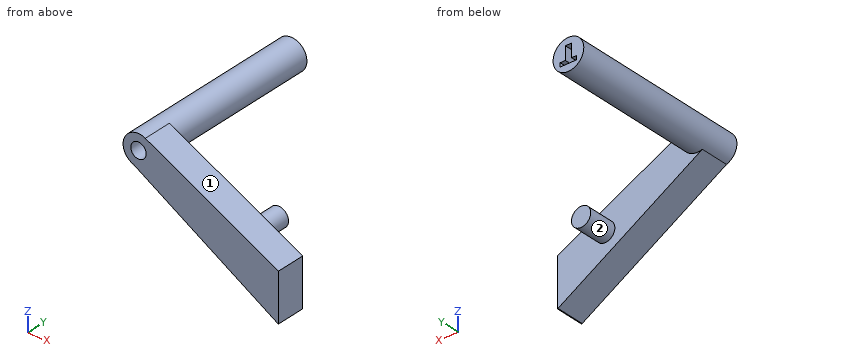
```python
from build123d import *

# Parameters (mm, degrees)
SKETCH1_R           = 8
BOSS_EXTRUDE1_DEPTH = 95
SKETCH2_R           = 4
CUT_EXTRUDE1_DEPTH  = 45
SKETCH3_W           = 8.60885167
SKETCH3_H           = 2.035138461
SKETCH3_W_2         = 3.196177608
SKETCH3_H_2         = 6.875388446
CUT_EXTRUDE2_DEPTH  = 40
BOSS_EXTRUDE2_DEPTH = 15
SKETCH5_R           = 5
BOSS_EXTRUDE3_DEPTH = 15


with BuildPart() as part:
    # Sketch1 → Boss-Extrude1 (new body)
    with BuildSketch(Plane(origin=(0, 0, 0), x_dir=(1, 0, 0), z_dir=(0, 1, 0))):
        with Locations(Location((0, 0, 0), (0, 0, 270))):
            Circle(SKETCH1_R)
    extrude(amount=BOSS_EXTRUDE1_DEPTH)

    # Sketch2 → Cut-Extrude1 (cut)
    with BuildSketch(Plane.XZ):
        with Locations(Location((0, 0, 0), (0, 0, 270))):
            Circle(SKETCH2_R)
    extrude(amount=-CUT_EXTRUDE1_DEPTH, mode=Mode.SUBTRACT)

    # Sketch3 → Cut-Extrude2 (cut)
    with BuildSketch(Plane(origin=(0, 95, 0), x_dir=(1, 0, 0), z_dir=(0, 1, 0))):
        with Locations((0, 3.24887213)):
            Rectangle(SKETCH3_W, SKETCH3_H)
        with Locations((0, -1.206391324)):
            Rectangle(SKETCH3_W_2, SKETCH3_H_2)
    extrude(amount=-CUT_EXTRUDE2_DEPTH, mode=Mode.SUBTRACT)

    # Sketch4 → Boss-Extrude2 (add)
    with BuildSketch(Plane.XZ):
        with BuildLine():
            ThreePointArc((72.61474538, -52.266719107), (72.807969556, -52.302734502), (73.001736138, -52.33570725))
            Line((73.001736138, -52.33570725), (73.001736138, -27.496744571))
            Line((73.001736138, -27.496744571), (3.57279106, 7.157874268))
            ThreePointArc((3.57279106, 7.157874268), (7.382913261, -3.081004996), (-2.575137965, -7.574210484))
            Line((-2.575137965, -7.574210484), (72.61474538, -52.266719107))
        make_face()
    extrude(amount=-BOSS_EXTRUDE2_DEPTH)

    # Sketch5 → Boss-Extrude3 (add)
    with BuildSketch(Plane(origin=(0, 15, 0), x_dir=(1, 0, 0), z_dir=(0, 1, 0))):
        with Locations(Location((48.001736138, 26.246610631, 0), (0, 0, 90))):
            Circle(SKETCH5_R)
    extrude(amount=BOSS_EXTRUDE3_DEPTH)

    # Sketch9 → Cut-Revolve2 (revolve, cut)
    with BuildSketch(Plane(origin=(0, 0, 0), x_dir=(0.6901743919423456, 0, -0.7236430810192366), z_dir=(-0.7236430810192366, 0, -0.6901743919423456)), mode=Mode.PRIVATE) as cut_revolve2_sk:
        Polygon((-4, -45), (0, -45), (0, -51.92820323), align=None)
    revolve(cut_revolve2_sk.sketch.rotate(Axis((0, 45, 0), (0, 1, 0)), 242.42131363), axis=Axis((0, 45, 0), (0, 1, 0)), mode=Mode.SUBTRACT)


solid = part.part
```
Geometry check sheet. Reference: the model listing, model coordinates, mm. Face numbers are marked on the shaded views. A direction names the side the tool comes from. Give positions to 0.01 mm unless a question says otherwise; leave off trailing zeros. Write each loop counter-clockwise with the first axis right and the second up, starting at its lowest first coordinate (ties: lowest second). Pieces come first, ordered by that corner, then holes. Notation, with made-up numbers: (38.25, -19.75) - (80.25, -19.75) arc R13 cw to (80.25, -1.75) - close; hole circle Ø9 at (85.5, 71.25). An arc over 180 degrees is marked (long way). Use a Markdown table: item, result.
Q1. Section check C-C, the plane x = 28.5. Enter the section's corners in (y, z), then the cut area to 3 significant figures.
Computed:
| item | result |
|---|---|
| outline | (0, -26.05) - (15, -26.05) - (15, -5.28) - (0, -5.28) - close |
| area | 311 mm² |
Q2. Go/stop test with flat-tipped pins: P1, Ø2, axis at x = 38.5, z = -11.5, coming from the +Y side; P2, Ø11, axis at x = 46, z = -27, coming from the +Y side; P3, Ø1.6, axis at y = 71, z = -3, coming from the -X side. Record where each tip stops, or that it passes through.
Computed:
| item | result |
|---|---|
| P1 | stops at y = 15 |
| P2 | stops at y = 30 |
| P3 | stops at x = -7.69 |
Q3. Section check D-D, the plane z = -20. Enter the section's corners in (x, y), then the cut area to 3 significant figures.
Computed:
| item | result |
|---|---|
| outline | (18.33, 0) - (57.98, 0) - (57.98, 15) - (18.33, 15) - close |
| area | 595 mm² |
Q4. Section check A-A, the plane y = 79. Enter the section's corners in (x, z).
Computed:
| item | result |
|---|---|
| outline | circle Ø16 at (0, 0); hole (-4.3, -4.27) - (4.3, -4.27) - (4.3, -2.23) - (1.6, -2.23) - (1.6, 4.64) - (-1.6, 4.64) - (-1.6, -2.23) - (-4.3, -2.23) - close |
Q5. Section check B-B, the plane y = 11. Enter the section's corners in (x, z).
Computed:
| item | result |
|---|---|
| outline | (-2.58, -7.57) - (72.61, -52.27) arc R12.5 ccw to (73, -52.34) - (73, -27.5) - (3.57, 7.16) arc R8 ccw (long way) to start; hole circle Ø8 at (0, 0) |
Q6. Thickness scan on L1, parallel to Z at x = 0, y = 18; L2, parallel to Y at x = 61.5, z = -37. Record the ranges inside material, lowest first. Write a range as [from, to].
Computed:
| item | result |
|---|---|
| L1 | z = [-8, -4], [4, 8] |
| L2 | y = [0, 15] |
Q7. Set-up check for the marked faces 1 and 2: record each of +Z, -Z, +X, -X, +Y, -Y from which the full face is reachable in a straight line by a thin tool's end or side.
Computed:
| item | result |
|---|---|
| face 1 | +Z, +X, +Y, -Y |
| face 2 | +Y |
